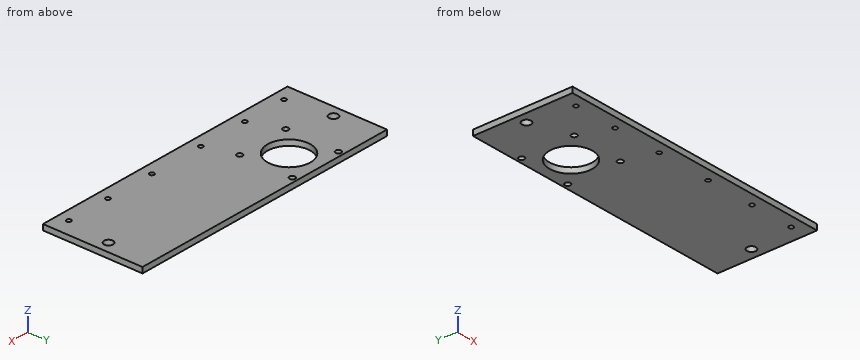
from build123d import *

# Parameters (mm, degrees)
SKIZZE1_W                       = 250
SKIZZE1_H                       = 89.2
AUFSATZ_LINEAR_AUSTRAGEN1_DEPTH = 5
SKIZZE2_R                       = 19.0625
SCHNITT_LINEAR_AUSTRAGEN1_DEPTH = 27
SKIZZE3_R                       = 2
SCHNITT_LINEAR_AUSTRAGEN2_DEPTH = 10
SKIZZE4_R                       = 4
SCHNITT_LINEAR_AUSTRAGEN3_DEPTH = 10
SKIZZE5_R                       = 2.5
SCHNITT_LINEAR_AUSTRAGEN4_DEPTH = 10
SKIZZE6_R                       = 2
SCHNITT_LINEAR_AUSTRAGEN5_DEPTH = 10


with BuildPart() as part:
    # Skizze1 → Aufsatz-Linear austragen1 (new body)
    with BuildSketch(Plane.XY):
        with Locations((125, 44.6)):
            Rectangle(SKIZZE1_W, SKIZZE1_H)
    extrude(amount=-AUFSATZ_LINEAR_AUSTRAGEN1_DEPTH)

    # Skizze2 → Schnitt-Linear austragen1 (cut)
    with BuildSketch(Plane.XY):
        with Locations((68, 61)):
            Circle(SKIZZE2_R)
    extrude(amount=-SCHNITT_LINEAR_AUSTRAGEN1_DEPTH, mode=Mode.SUBTRACT)

    # Skizze3 → Schnitt-Linear austragen2 (cut)
    with BuildSketch(Plane.XY):
        with Locations((15, 10)):
            Circle(SKIZZE3_R)
        with Locations((55, 10)):
            Circle(SKIZZE3_R)
        with Locations((195, 10)):
            Circle(SKIZZE3_R)
        with Locations((235, 10)):
            Circle(SKIZZE3_R)
        with Locations((150, 10)):
            Circle(SKIZZE3_R)
    extrude(amount=-SCHNITT_LINEAR_AUSTRAGEN2_DEPTH, mode=Mode.SUBTRACT)

    # Skizze4 → Schnitt-Linear austragen3 (cut)
    with BuildSketch(Plane.XY):
        with Locations((10, 50)):
            Circle(SKIZZE4_R)
        with Locations((240, 50)):
            Circle(SKIZZE4_R)
    extrude(amount=-SCHNITT_LINEAR_AUSTRAGEN3_DEPTH, mode=Mode.SUBTRACT)

    # Skizze5 → Schnitt-Linear austragen4 (cut)
    with BuildSketch(Plane.XY):
        with Locations((44.43, 84.57)):
            Circle(SKIZZE5_R)
        with Locations((91.57, 84.57)):
            Circle(SKIZZE5_R)
        with Locations((91.57, 37.43)):
            Circle(SKIZZE5_R)
        with Locations((44.43, 37.43)):
            Circle(SKIZZE5_R)
    extrude(amount=-SCHNITT_LINEAR_AUSTRAGEN4_DEPTH, mode=Mode.SUBTRACT)

    # Skizze6 → Schnitt-Linear austragen5 (cut)
    with BuildSketch(Plane.XY):
        with Locations((100, 10)):
            Circle(SKIZZE6_R)
    extrude(amount=-SCHNITT_LINEAR_AUSTRAGEN5_DEPTH, mode=Mode.SUBTRACT)


solid = part.part
Can you work these out from the model? Positions are in its coordinate system, mm. Round coordinates to 2 decimals unless told otherwise and drop trailing zeros. Order: outer loops, then holes, each group sorted by start corner. A loop starts at its lowest first (then second) coordinate and runs counter-clockwise, first axis right, second up. Notation, with made-up numbers: M 67.25,74 L 76.25,74 A18 cw 76.25,104 Z; hole C 40.5,-17.75 d7. An arc over 180 degrees is marked long. Use a Markdown table: item, result.
1) Imagine slicing it at B-B (z = -1). Give the number of separate pieces and of enclosed holes in the cut face, then the cut area to 3 significant figures.
Geometry says:
| item | result |
|---|---|
| separate pieces | 1 |
| enclosed holes | 13 |
| area | 20,900 mm² |
2) If I drill on line 1 along Y through (x, z) = (44.43, -3.9); line 2 along Y through (x, z) = (93.5, -2.4); line 3 along Y through (x, z) = (100, -3), over which ranges is the centre line in solid material (lowest first)?
Geometry says:
| item | result |
|---|---|
| line 1 | y = 0 to 34.93, 39.93 to 82.07, 87.07 to 89.2 |
| line 2 | y = 0 to 35.84, 39.02 to 82.98, 86.16 to 89.2 |
| line 3 | y = 0 to 8, 12 to 89.2 |
3) Imagine slicing it at C-C (x = 10). List the corners of the cut face in (y, z) for me.
Geometry says:
| item | result |
|---|---|
| outline | M 0,-5 L 46,-5 L 46,0 L 0,0 Z; M 54,-5 L 89.2,-5 L 89.2,0 L 54,0 Z |
4) Imagine slicing it at A-A (x = 68). List the corners of the cut face in (y, z) for me, then the cut area to 3 significant figures.
Geometry says:
| item | result |
|---|---|
| outline | M 0,-5 L 41.94,-5 L 41.94,0 L 0,0 Z; M 80.06,-5 L 89.2,-5 L 89.2,0 L 80.06,0 Z |
| area | 255 mm² |
5) I'm going to push a flat-ended pin straight in: P1, Ø7, axis at x = 10, y = 50, coming from the -Z side. Where does the tip first touch, or does it pass through?
Geometry says:
| item | result |
|---|---|
| P1 | passes through |
